```python
from build123d import *

# Parameters (mm, degrees)
SKETCH1_R           = 5
SKETCH1_R_2         = 3
BOSS_EXTRUDE2_DEPTH = 17.5
SKETCH4_W           = 18
SKETCH4_H           = 1
EXTRUDE_THIN1_DEPTH = 35
CIRPATTERN1_COUNT   = 9
SKETCH5_R           = 3
BOSS_EXTRUDE3_DEPTH = 15
SKETCH6_R           = 3.5
SKETCH6_R_2         = 1.5
CUT_EXTRUDE1_DEPTH  = 6
SKETCH15_R          = 1.5
CUT_EXTRUDE2_DEPTH  = 2
SKETCH17_R          = 2.5
BOSS_EXTRUDE4_DEPTH = 3
SKETCH18_R          = 2
CUT_EXTRUDE3_DEPTH  = 2
SKETCH19_R          = 4
CUT_EXTRUDE4_DEPTH  = 20
SKETCH20_W          = 45.677284088
SKETCH20_H          = 45.724664858
CUT_EXTRUDE5_DEPTH  = 8
SKETCH21_R          = 3
BOSS_EXTRUDE5_DEPTH = 1
SKETCH24_R          = 9.912143672
BOSS_EXTRUDE6_DEPTH = 0.5
SKETCH25_R          = 3.2
CUT_EXTRUDE6_DEPTH  = 2.1
SKETCH26_R          = 3.2
BOSS_EXTRUDE7_DEPTH = 0.25
CUT_EXTRUDE8_START  = -7.5
CUT_EXTRUDE8_DEPTH  = 7.5
SKETCH28_R          = 0.5
CUT_EXTRUDE9_DEPTH  = 1.5
CUT_EXTRUDE10_DEPTH = 7
BOSS_EXTRUDE8_START = 10
SKETCH30_R          = 4
BOSS_EXTRUDE8_DEPTH = 10
SKETCH33_R          = 18.064901356
CUT_EXTRUDE13_DEPTH = 20
SKETCH34_R          = 3
CUT_EXTRUDE14_DEPTH = 8.5
SKETCH35_R          = 0.75
CUT_EXTRUDE16_DEPTH = 3


with BuildPart() as part:
    # Sketch1 → Boss-Extrude2 (new, symmetric)
    with BuildSketch(Plane(origin=(0, 0, 0), x_dir=(1, 0, 0), z_dir=(0, 1, 0))):
        with Locations(Location((0, 0, 0), (0, 0, 270))):
            Circle(SKETCH1_R)
        with Locations(Location((0, 0, 0), (0, 0, 270))):
            Circle(SKETCH1_R_2, mode=Mode.SUBTRACT)
    extrude(amount=BOSS_EXTRUDE2_DEPTH, both=True)

    # Sketch4 → Extrude-Thin1 (add)
    with BuildSketch(Plane(origin=(0, 17.5, 0), x_dir=(1, 0, 0), z_dir=(0, 1, 0))):
        with Locations((12, 0)):
            Rectangle(SKETCH4_W, SKETCH4_H)
    extrude_thin1 = extrude(amount=-EXTRUDE_THIN1_DEPTH)

    # CirPattern1: Extrude-Thin1 ×9 about axis
    cirpattern1_axis = Axis((0, 0, 0), (0, 1, 0))
    for i in range(1, CIRPATTERN1_COUNT):
        add(extrude_thin1.rotate(cirpattern1_axis, i * 360 / CIRPATTERN1_COUNT))

    # Sketch5 → Boss-Extrude3 (add)
    with BuildSketch(Plane(origin=(0, -17.5, 0), x_dir=(-1, 0, 0), z_dir=(0, -1, 0))):
        with Locations(Location((0, 0, 0), (0, 0, 90))):
            Circle(SKETCH5_R)
    extrude(amount=-BOSS_EXTRUDE3_DEPTH)

    # Sketch6 → Cut-Extrude1 (cut)
    with BuildSketch(Plane(origin=(0, -17.5, 0), x_dir=(-1, 0, 0), z_dir=(0, -1, 0))):
        with Locations(Location((0, 0, 0), (0, 0, 90))):
            Circle(SKETCH6_R)
        with Locations(Location((0, 0, 0), (0, 0, 90))):
            Circle(SKETCH6_R_2, mode=Mode.SUBTRACT)
    extrude(amount=-CUT_EXTRUDE1_DEPTH, mode=Mode.SUBTRACT)

    # Sketch15 → Cut-Extrude2 (cut)
    with BuildSketch(Plane.XZ.offset(17.5)):
        with Locations(Location((0, 0, 0), (0, 0, 270))):
            Circle(SKETCH15_R)
    extrude(amount=-CUT_EXTRUDE2_DEPTH, mode=Mode.SUBTRACT)

    # Sketch17 → Boss-Extrude4 (add)
    with BuildSketch(Plane.XZ.offset(17.5)):
        with Locations((18.5, 0)):
            Circle(SKETCH17_R)
    extrude(amount=-BOSS_EXTRUDE4_DEPTH)

    # Sketch18 → Cut-Extrude3 (cut)
    with BuildSketch(Plane.XZ.offset(17.5)):
        with Locations(Location((18.5, 0, 0), (0, 0, 270))):
            Circle(SKETCH18_R)
    extrude(amount=-CUT_EXTRUDE3_DEPTH, mode=Mode.SUBTRACT)

    # Sketch19 → Cut-Extrude4 (cut)
    with BuildSketch(Plane(origin=(0, 17.5, 0), x_dir=(1, 0, 0), z_dir=(0, 1, 0))):
        with Locations(Location((0, 0, 0), (0, 0, 270))):
            Circle(SKETCH19_R)
    extrude(amount=-CUT_EXTRUDE4_DEPTH, mode=Mode.SUBTRACT)

    # Sketch20 → Cut-Extrude5 (cut)
    with BuildSketch(Plane(origin=(0, -17.5, 0), x_dir=(-1, 0, 0), z_dir=(0, -1, 0))):
        Rectangle(SKETCH20_W, SKETCH20_H)
    extrude(amount=-CUT_EXTRUDE5_DEPTH, mode=Mode.SUBTRACT)

    # Sketch21 → Boss-Extrude5 (add)
    with BuildSketch(Plane.XZ.offset(9.5)):
        with Locations(Location((0, 0, 0), (0, 0, 90))):
            Circle(SKETCH21_R)
    extrude(amount=BOSS_EXTRUDE5_DEPTH)

    # Sketch23 → Revolve1 (revolve)
    with BuildSketch(Plane(origin=(0, 0, 0), x_dir=(0, 0, -1), z_dir=(1, 0, 0))):
        with BuildLine():
            Line((-3, -10.5), (-2, -10.5))
            Line((-2, -10.5), (0, -10.5))
            Line((0, -10.5), (0, -17.5))
            Line((0, -17.5), (-8.912143672, -17.5))
            Line((-8.912143672, -17.5), (-9.912143672, -17.5))
            ThreePointArc((-9.912143672, -17.5), (-7.260403323, -13.2057636), (-3, -10.5))
        make_face()
    revolve(axis=Axis((0, -11.130650603, 0), (0, -1, 0)))

    # Sketch24 → Boss-Extrude6 (add)
    with BuildSketch(Plane.XZ.offset(17.5)):
        with Locations(Location((0, 0, 0), (0, 0, 270))):
            Circle(SKETCH24_R)
    extrude(amount=BOSS_EXTRUDE6_DEPTH)

    # Sketch25 → Cut-Extrude6 (cut)
    with BuildSketch(Plane.XZ.offset(18)):
        with Locations(Location((-0.56668442, 5, 0), (0, 0, 270))):
            Circle(SKETCH25_R)
    extrude(amount=-CUT_EXTRUDE6_DEPTH, mode=Mode.SUBTRACT)

    # Sketch26 → Boss-Extrude7 (add)
    with BuildSketch(Plane.XZ.offset(18)):
        with Locations(Location((-0.56668442, 5, 0), (0, 0, 270))):
            Circle(SKETCH26_R)
    extrude(amount=-BOSS_EXTRUDE7_DEPTH)

    # Sketch27 → Cut-Extrude8 (cut)
    with BuildSketch(Plane.XZ.offset(18).offset(CUT_EXTRUDE8_START)):
        with BuildLine():
            ThreePointArc((-5.368630905, 4.991892601), (-6.424807204, 5.779358473), (-7.613826501, 6.346671425))
            ThreePointArc((-7.613826501, 6.346671425), (-9.912143672, 0), (-7.613826501, -6.346671425))
            ThreePointArc((-7.613826501, -6.346671425), (-6.424807204, -5.779358473), (-5.368630905, -4.991892601))
            ThreePointArc((-5.368630905, -4.991892601), (-3.162143672, 0), (-5.368630905, 4.991892601))
        make_face()
        with BuildLine():
            ThreePointArc((9.912143672, 0), (9.319869483, 3.375), (7.613826501, 6.346671425))
            ThreePointArc((7.613826501, 6.346671425), (6.424807204, 5.779358473), (5.368630905, 4.991892601))
            ThreePointArc((5.368630905, 4.991892601), (3.162143672, 0), (5.368630905, -4.991892601))
            ThreePointArc((5.368630905, -4.991892601), (6.424807204, -5.779358473), (7.613826501, -6.346671425))
            ThreePointArc((7.613826501, -6.346671425), (9.319869483, -3.375), (9.912143672, 0))
        make_face()
        with BuildLine():
            ThreePointArc((-5.368630905, -4.991892601), (-6.424807204, -5.779358473), (-7.613826501, -6.346671425))
            ThreePointArc((-7.613826501, -6.346671425), (-4.203657524, -8.976628297), (0, -9.912143672))
            add(Edge.make_bspline(
                [(-5.368630905, -4.991892601), (-4.998119196, -7.539682857), (-2.616364035, -9.837937814), (0, -9.912143672)],
                knots=[0, 0, 0, 0, 1, 1, 1, 1], degree=3))
        make_face()
        with BuildLine():
            add(Edge.make_bspline(
                [(5.368630905, -4.991892601), (4.998119196, -7.539682857), (2.616364035, -9.837937814), (0, -9.912143672)],
                knots=[0, 0, 0, 0, 1, 1, 1, 1], degree=3))
            ThreePointArc((0, -9.912143672), (4.203657524, -8.976628297), (7.613826501, -6.346671425))
            ThreePointArc((7.613826501, -6.346671425), (6.424807204, -5.779358473), (5.368630905, -4.991892601))
        make_face()
        with BuildLine():
            ThreePointArc((0, 9.912143672), (-4.203657524, 8.976628297), (-7.613826501, 6.346671425))
            ThreePointArc((-7.613826501, 6.346671425), (-6.424807204, 5.779358473), (-5.368630905, 4.991892601))
            add(Edge.make_bspline(
                [(-5.368630905, 4.991892601), (-4.998119196, 7.539682857), (-2.616364035, 9.837937814), (0, 9.912143672)],
                knots=[0, 0, 0, 0, 1, 1, 1, 1], degree=3))
        make_face()
        with BuildLine():
            ThreePointArc((7.613826501, 6.346671425), (4.203657524, 8.976628297), (0, 9.912143672))
            add(Edge.make_bspline(
                [(5.368630905, 4.991892601), (4.998119196, 7.539682857), (2.616364035, 9.837937814), (0, 9.912143672)],
                knots=[0, 0, 0, 0, 1, 1, 1, 1], degree=3))
            ThreePointArc((5.368630905, 4.991892601), (6.424807204, 5.779358473), (7.613826501, 6.346671425))
        make_face()
    extrude(amount=CUT_EXTRUDE8_DEPTH, mode=Mode.SUBTRACT)

    # Sketch28 → Cut-Extrude9 (cut)
    with BuildSketch(Plane.XZ.offset(18)):
        with Locations(Location((0, 0, 0), (0, 0, 270))):
            Circle(SKETCH28_R)
    extrude(amount=-CUT_EXTRUDE9_DEPTH, mode=Mode.SUBTRACT)

    # Sketch29 → Cut-Extrude10 (cut)
    with BuildSketch(Plane(origin=(0, 17.5, 0), x_dir=(1, 0, 0), z_dir=(0, 1, 0))):
        with BuildLine():
            Line((3.489629181, -3.580850203), (15.765539501, -13.881562025))
            Line((15.765539501, -13.881562025), (16.40832711, -13.115517582))
            Line((16.40832711, -13.115517582), (4.132416791, -2.81480576))
            ThreePointArc((4.132416791, -2.81480576), (4.698463104, -1.710100717), (4.974937186, -0.5))
            Line((4.974937186, -0.5), (21, -0.5))
            Line((21, -0.5), (21, 0.5))
            Line((21, 0.5), (4.974937186, 0.5))
            ThreePointArc((4.974937186, 0.5), (4.698463104, 1.710100717), (4.132416791, 2.81480576))
            Line((4.132416791, 2.81480576), (16.40832711, 13.115517582))
            Line((16.40832711, 13.115517582), (15.765539501, 13.881562025))
            Line((15.765539501, 13.881562025), (3.489629181, 3.580850203))
            ThreePointArc((3.489629181, 3.580850203), (2.5, 4.330127019), (1.356292653, 4.812532622))
            Line((1.356292653, 4.812532622), (4.139015608, 20.594138724))
            Line((4.139015608, 20.594138724), (3.154207854, 20.767786902))
            Line((3.154207854, 20.767786902), (0.3714849, 4.9861808))
            ThreePointArc((0.3714849, 4.9861808), (-0.868240888, 4.924038765), (-2.054455891, 4.558421985))
            Line((-2.054455891, 4.558421985), (-10.066987298, 18.436533479))
            Line((-10.066987298, 18.436533479), (-10.933012702, 17.936533479))
            Line((-10.933012702, 17.936533479), (-2.920481295, 4.058421985))
            ThreePointArc((-2.920481295, 4.058421985), (-3.830222216, 3.213938048), (-4.50390169, 2.17137504))
            Line((-4.50390169, 2.17137504), (-19.562534965, 7.65226932))
            Line((-19.562534965, 7.65226932), (-19.904555108, 6.712576699))
            Line((-19.904555108, 6.712576699), (-4.845921834, 1.231682419))
            ThreePointArc((-4.845921834, 1.231682419), (-5, 0), (-4.845921834, -1.231682419))
            Line((-4.845921834, -1.231682419), (-19.904555108, -6.712576699))
            Line((-19.904555108, -6.712576699), (-19.562534965, -7.65226932))
            Line((-19.562534965, -7.65226932), (-4.50390169, -2.17137504))
            ThreePointArc((-4.50390169, -2.17137504), (-3.830222216, -3.213938048), (-2.920481295, -4.058421985))
            Line((-2.920481295, -4.058421985), (-10.933012702, -17.936533479))
            Line((-10.933012702, -17.936533479), (-10.066987298, -18.436533479))
            Line((-10.066987298, -18.436533479), (-2.054455891, -4.558421985))
            ThreePointArc((-2.054455891, -4.558421985), (-0.868240888, -4.924038765), (0.3714849, -4.9861808))
            Line((0.3714849, -4.9861808), (3.154207854, -20.767786902))
            Line((3.154207854, -20.767786902), (4.139015608, -20.594138724))
            Line((4.139015608, -20.594138724), (1.356292653, -4.812532622))
            ThreePointArc((1.356292653, -4.812532622), (2.5, -4.330127019), (3.489629181, -3.580850203))
        make_face()
    extrude(amount=-CUT_EXTRUDE10_DEPTH, mode=Mode.SUBTRACT)

    # Sketch30 → Boss-Extrude8 (add)
    with BuildSketch(Plane(origin=(0, -2.5, 0), x_dir=(1, 0, 0), z_dir=(0, 1, 0)).offset(BOSS_EXTRUDE8_START)):
        with Locations(Location((0, 0, 0), (0, 0, 270))):
            Circle(SKETCH30_R)
    extrude(amount=-BOSS_EXTRUDE8_DEPTH)

    # Sketch33 → Cut-Extrude13 (cut)
    with BuildSketch(Plane.XZ.offset(9.5)):
        Circle(SKETCH33_R)
    extrude(amount=CUT_EXTRUDE13_DEPTH, mode=Mode.SUBTRACT)

    # Sketch34 → Cut-Extrude14 (cut)
    with BuildSketch(Plane.XZ.offset(9.5)):
        with Locations(Location((0, 0, 0), (0, 0, 270))):
            Circle(SKETCH34_R)
    extrude(amount=-CUT_EXTRUDE14_DEPTH, mode=Mode.SUBTRACT)

    # Sketch35 → Cut-Extrude16 (cut)
    with BuildSketch(Plane(origin=(0, 7.5, 0), x_dir=(1, 0, 0), z_dir=(0, 1, 0))):
        with Locations(Location((0, 0, 0), (0, 0, 270))):
            Circle(SKETCH35_R)
    extrude(amount=-CUT_EXTRUDE16_DEPTH, mode=Mode.SUBTRACT)


solid = part.part
```
Geometry check sheet. Reference: the model listing, model coordinates, mm. A direction names the side the tool comes from. Give positions to 0.01 mm unless a question says otherwise; leave off trailing zeros. Order: outer loops, then holes, each group sorted by start corner. A loop starts at its lowest first (then second) coordinate and runs counter-clockwise, first axis right, second up.
1. Section check C-C, the plane x = 12. Enter the section's corners in (y, z).
2. Section check A-A, the plane z = -17. Enter the section's corners in (x, y).
3. Thickness scan on L1, parallel to X at y = 8.25, z = 0; L2, parallel to Z at x = 5, y = -8.25; L3, parallel to X at y = -5.25, z = 0. Record the ranges inside material, lowest first.
4. Section check D-D, the plane z = -11. Enter the section's corners in (x, y), and give its area (3 significant figures).
5. Section check B-B, the plane x = -13. Enter the section's corners in (y, z).
6. Gauge pin test, flat ends, axial feed: pin 1 Ø5 at (x, y) = (17, 4) entering from -Z; pin 2 Ø4 at (x, z) = (1.5, -1) entering from +Y; pin 3 Ø3 at (x, z) = (-1, -2.5) entering from -Y; pin 4 Ø1 at (x, y) = (12.5, -6.5) entering from +Z. Record the tip position at first contact, or that the pin passes through.
7. Release check for a two-part mould opening along Z. For faces 1 (the face through (10.18, 0.64, 7.89)), 2 (the face through (3, 10.5, 3)), 3 (the face through (-19.736, 0.64, 7.176)), 4 (the face through (2.48, 0.64, 4.34)) record: pulls with the +Z half, pulls with the -Z half, needs draft (parallel to the pull), parting line crosses it, or undercut.
8. Access from +Z, -Z, +X, -X, +Y, -Y to the whole of each face (thin tool, end or side, straight path). Record for faces 5 (the face through (-6.005, 0.64, -11.4)), 6 (the face through (1.743, 0.64, 12.767)), 7 (the face through (-4, 1, -3)), 8 (the face through (13, 1, 0.5)), 9 (the face through (0, 4.5, 0)).
Values follow:
1. outline: (-9.5, -10.72) - (10.5, -10.72) - (10.5, -9.42) - (-9.5, -9.42) - close; (-9.5, -0.5) - (10.5, -0.5) - (10.5, 0.5) - (-9.5, 0.5) - close; (-9.5, 9.42) - (10.5, 9.42) - (10.5, 10.72) - (-9.5, 10.72) - close
2. outline: (-10.39, -9.5) - (-9.24, -9.5) - (-9.24, 10.5) - (-10.39, 10.5) - close; (2.49, -9.5) - (3.51, -9.5) - (3.51, 10.5) - (2.49, 10.5) - close
3. L1: x = -5 to -4, 4 to 21
3. L2: z = -4.85 to -3.54, -0.5 to 0.5, 3.54 to 4.85
3. L3: x = -5 to -3, 3 to 21
4. outline: (-6.93, -9.5) - (-5.77, -9.5) - (-5.77, 10.5) - (-6.93, 10.5) - close; (1.43, -9.5) - (2.45, -9.5) - (2.45, 10.5) - (1.43, 10.5) - close; (12.33, -9.5) - (13.89, -9.5) - (13.89, 10.5) - (12.33, 10.5) - close
4. area: 74.5 mm2
5. outline: (-9.5, -5.26) - (10.5, -5.26) - (10.5, -4.2) - (-9.5, -4.2) - close; (-9.5, 4.2) - (10.5, 4.2) - (10.5, 5.26) - (-9.5, 5.26) - close
6. pin 1: stops at z = -13.88
6. pin 2: stops at y = 7.5
6. pin 3: stops at y = -9.5
6. pin 4: stops at z = 11.56
7. face 1: undercut
7. face 2: needs draft
7. face 3: pulls with the +Z half
7. face 4: undercut
8. face 5: -Z, +Y, -Y
8. face 6: +Z, +Y, -Y
8. face 7: +Y, -Y
8. face 8: +X, +Y, -Y
8. face 9: +Y
